Could you check a few things on this drawing? It's one solid part, dimensions in mm from its lowest x, y, z. A direction names the side the tool comes from. Coordinates: 2 decimals unless noted, no trailing zeros. Write each loop counter-clockwise with the first axis right and the second up, starting at its lowest first coordinate (ties: lowest second). Pieces come first, ordered by that corner, then holes. Notation, with made-up numbers: M 75.5,50 L 131.5,50 A16 cw 131.5,58 Z; hole C -9.5,67 d5. An arc over 180 degrees is marked long. Use a Markdown table: item, result.
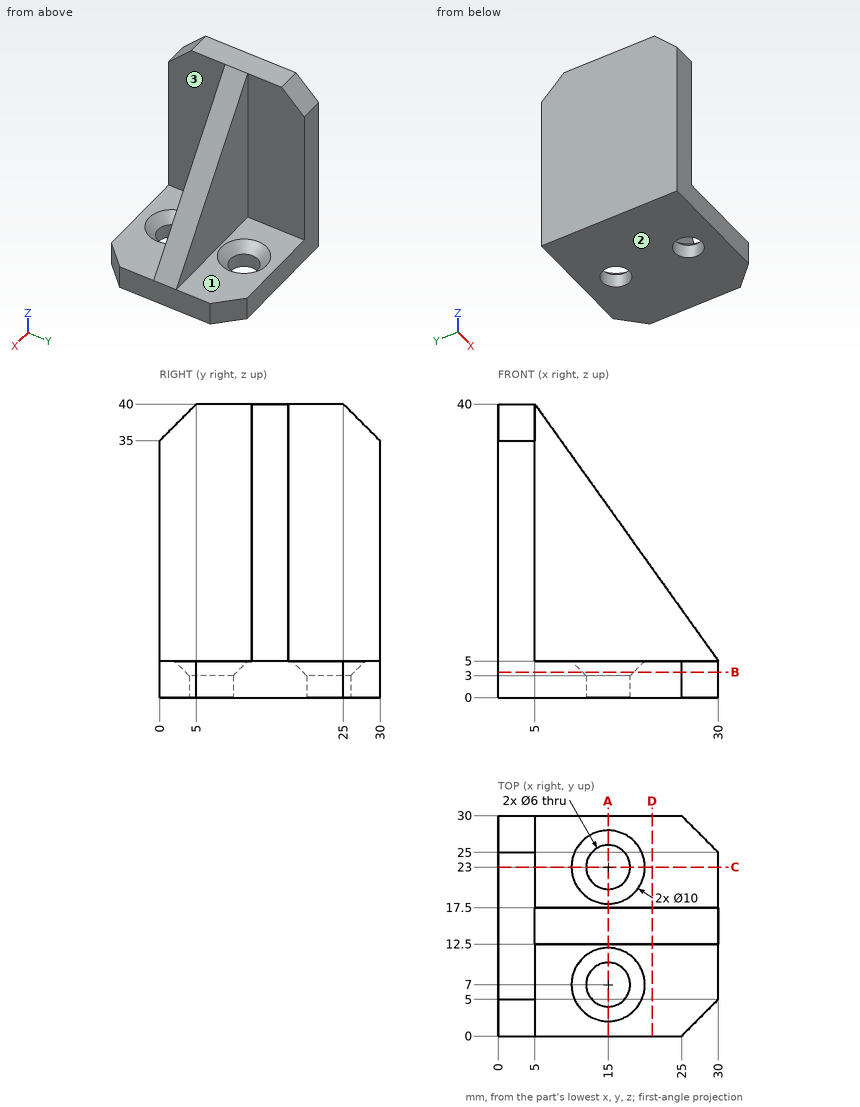
1. Which directions (+Z, -Z, +X, -X, +Y, -Y) give clear straight access to the entire face, cutting with the end or side of a thin tool? Please do the marked faces 1, 2 and 3.
Answers follow:
| item | result |
|---|---|
| face 1 | +Z, +X, +Y |
| face 2 | -Z, +X, -X, +Y, -Y |
| face 3 | +Z, +X, -Y |
2. Suppose I cut it at A-A on x = 15. Write out the boundary of the cut face in (y, z).
Answers follow:
| item | result |
|---|---|
| outline | M 0,0 L 4,0 L 4,3 L 2,5 L 0,5 Z; M 10,0 L 20,0 L 20,3 L 18,5 L 17.5,5 L 17.5,26 L 12.5,26 L 12.5,5 L 12,5 L 10,3 Z; M 26,0 L 30,0 L 30,5 L 28,5 L 26,3 Z |
3. Suppose I cut it at D-D on x = 21. Write out the boundary of the cut face in (y, z), and give its area (3 significant figures).
Answers follow:
| item | result |
|---|---|
| outline | M 0,0 L 30,0 L 30,5 L 17.5,5 L 17.5,17.6 L 12.5,17.6 L 12.5,5 L 0,5 Z |
| area | 213 mm2 |
4. Suppose I cut it at C-C on y = 23. Write out the boundary of the cut face in (x, z), and give its area (3 significant figures).
Answers follow:
| item | result |
|---|---|
| outline | M 0,0 L 12,0 L 12,3 L 10,5 L 5,5 L 5,40 L 0,40 Z; M 18,0 L 30,0 L 30,5 L 20,5 L 18,3 Z |
| area | 291 mm2 |
5. Will these pins go through, and if not, where does the flat tip stop? pin 1 Ø1 at (x, y) = (15.5, 20) entering from +Z; pin 2 Ø6 at (x, y) = (26.5, 4.5) entering from +Z; pin 3 Ø7 at (x, y) = (15, 23) entering from -Z; pin 4 Ø1 at (x, z) = (13.5, 17) entering from +Y.
Answers follow:
| item | result |
|---|---|
| pin 1 | stops at z = 3.54 |
| pin 2 | stops at z = 5 |
| pin 3 | stops at z = 0 |
| pin 4 | stops at y = 17.5 |
6. Suppose I cut it at B-B on z = 3.5. Write out the boundary of the cut face in (x, y), and give its area (3 significant figures).
Answers follow:
| item | result |
|---|---|
| outline | M 0,0 L 25,0 L 30,5 L 30,25 L 25,30 L 0,30 Z; hole C 15,7 d7; hole C 15,23 d7 |
| area | 798 mm2 |
7. I need wall thicknesses on probe 1 along Y at (x, z) = (15, 1.7); probe 2 along Y at (x, z) = (18, 20); probe 3 along Z at (x, y) = (28, 5.5). Which ranges of each line are inside material? Lowest first, please.
Answers follow:
| item | result |
|---|---|
| probe 1 | y = 0 to 4, 10 to 20, 26 to 30 |
| probe 2 | y = 12.5 to 17.5 |
| probe 3 | z = 0 to 5 |
